For this review, take the finished solid that the model builds, in its own axes (mm). A direction names the side the tool comes from. Coordinates: 2 decimals unless noted, no trailing zeros. Loops run counter-clockwise (first coordinate to the right, second up) from the corner with the lowest first, then second, coordinate; pieces in that order, holes last. Notation, with made-up numbers: M -26,11 L -12,11 A21 cw -12,39 Z; hole C -18,-2 d8. An arc over 180 degrees is marked long. Put each result on its own line as item: value.
```python
from build123d import *

# Parameters (mm, degrees)
BOSS_EXTRUDE1_DEPTH = 1.1
SKETCH3_W           = 122
SKETCH3_H           = 254
BOSS_EXTRUDE2_DEPTH = 1
SKETCH4_W           = 32
SKETCH4_H           = 226
BOSS_EXTRUDE3_DEPTH = 10.6
SKETCH5_R           = 1.5
BOSS_EXTRUDE4_DEPTH = 30.1


with BuildPart() as part:
    # Sketch2 → Boss-Extrude1 (new body)
    with BuildSketch(Plane.XY):
        with BuildLine():
            Line((-76.67, -127.5), (76.67, -127.5))
            ThreePointArc((76.67, -127.5), (81.499539316, -125.499539316), (83.5, -120.67))
            Line((83.5, -120.67), (83.5, 120.67))
            ThreePointArc((83.5, 120.67), (81.499539316, 125.499539316), (76.67, 127.5))
            Line((76.67, 127.5), (-76.67, 127.5))
            ThreePointArc((-76.67, 127.5), (-81.499539316, 125.499539316), (-83.5, 120.67))
            Line((-83.5, 120.67), (-83.5, -120.67))
            ThreePointArc((-83.5, -120.67), (-81.499539316, -125.499539316), (-76.67, -127.5))
        make_face()
    extrude(amount=BOSS_EXTRUDE1_DEPTH)

    # Sketch3 → Boss-Extrude2 (add)
    with BuildSketch(Plane(origin=(0, 0, 0), x_dir=(-1, 0, 0), z_dir=(0, 0, -1))):
        with Locations((14.96, 0)):
            Rectangle(SKETCH3_W, SKETCH3_H)
    extrude(amount=BOSS_EXTRUDE2_DEPTH)

    # Sketch4 → Boss-Extrude3 (add)
    with BuildSketch(Plane(origin=(0, 0, 0), x_dir=(-1, 0, 0), z_dir=(0, 0, -1))):
        with Locations((-62.04, 0)):
            Rectangle(SKETCH4_W, SKETCH4_H)
    extrude(amount=BOSS_EXTRUDE3_DEPTH)

    # Sketch5 → Boss-Extrude4 (add)
    with BuildSketch(Plane(origin=(0, 0, 0), x_dir=(-1, 0, 0), z_dir=(0, 0, -1))):
        with Locations((-23.21, -104.9)):
            Circle(SKETCH5_R)
        with Locations((57.3, -104.9)):
            Circle(SKETCH5_R)
        with Locations((57.3, 104.9)):
            Circle(SKETCH5_R)
        with Locations((-23.21, 104.9)):
            Circle(SKETCH5_R)
    extrude(amount=BOSS_EXTRUDE4_DEPTH)


solid = part.part
```
(1) Wall thickness on line 1 along Z through (x, y) = (46, 4.5); line 2 along X through (y, z) = (-5.5, -9.5); line 3 along Z through (x, y) = (74, -84.5): over which ranges is each line inside the solid? List them lowest first. Write a range as [from, to].
Determined:
line 1: z = [-1, 1.1]
line 2: x = [46.04, 78.04]
line 3: z = [-10.6, 1.1]
(2) For pin 1 (3 mm diameter, centred on y = -38, z = -4.5, fed in from -X); pin 2 (5.5 mm diameter, centred on y = -7, z = -8, fed in from +X); pin 3 (1 mm diameter, centred on y = -23, z = -12, fed in from +X); pin 4 (1 mm diameter, centred on x = -3, y = 2.5, fed in from -Z), all flat-tipped, find the tip position at first contact; note any pin that passes through.
Determined:
pin 1: stops at x = 46.04
pin 2: stops at x = 78.04
pin 3: passes through
pin 4: stops at z = -1
(3) Tool access review of faces 1 (the flat face through (-1, 2, 1.1)), 2 (the flat face through (78.04, -2, -5)): name each direction out of +Z, -Z, +X, -X, +Y, -Y from which nothing blocks a thin tool from reaching the whole face with its end or side.
Determined:
face 1: +Z, +X, -X, +Y, -Y
face 2: -Z, +X, +Y, -Y
(4) Add section B-B (x = -36.5). Write out the cut boundary in (y, z), plus the area to 4 significant figures.
Determined:
outline: M -127.5,0 L -127,0 L -127,-1 L 127,-1 L 127,0 L 127.5,0 L 127.5,1.1 L -127.5,1.1 Z
area: 534.5 mm^2
(5) Add section C-C (y = -29). Write out the cut boundary in (x, z), plus the area to 3 significant figures.
Determined:
outline: M -83.5,0 L -75.96,0 L -75.96,-1 L 46.04,-1 L 46.04,-10.6 L 78.04,-10.6 L 78.04,0 L 83.5,0 L 83.5,1.1 L -83.5,1.1 Z
area: 645 mm^2
(6) Add section A-A (z = -6). Write out the cut boundary in (x, y).
Determined:
outline: C -57.3,-104.9 d3; C -57.3,104.9 d3; C 23.21,-104.9 d3; C 23.21,104.9 d3; M 46.04,-113 L 78.04,-113 L 78.04,113 L 46.04,113 Z
